Input: dimensioned drawing with shaded views. Units: mm. Origin: part minimum x, y, z. A direction names the side the tool comes from. Give positions to 0.01 mm unless a question says otherwise; leave off trailing zeros. Order: outer loops, then holes, each group sorted by start corner. A loop starts at its lowest first (then second) coordinate and runs counter-clockwise, first axis right, second up. Notation, with made-up numbers: (6, 71) - (55, 71) arc R14 ccw to (55, 85) - close; hole circle Ø1 at (9, 28.5). An arc over 180 degrees is marked (long way). Answer as CSV lines item,"result".
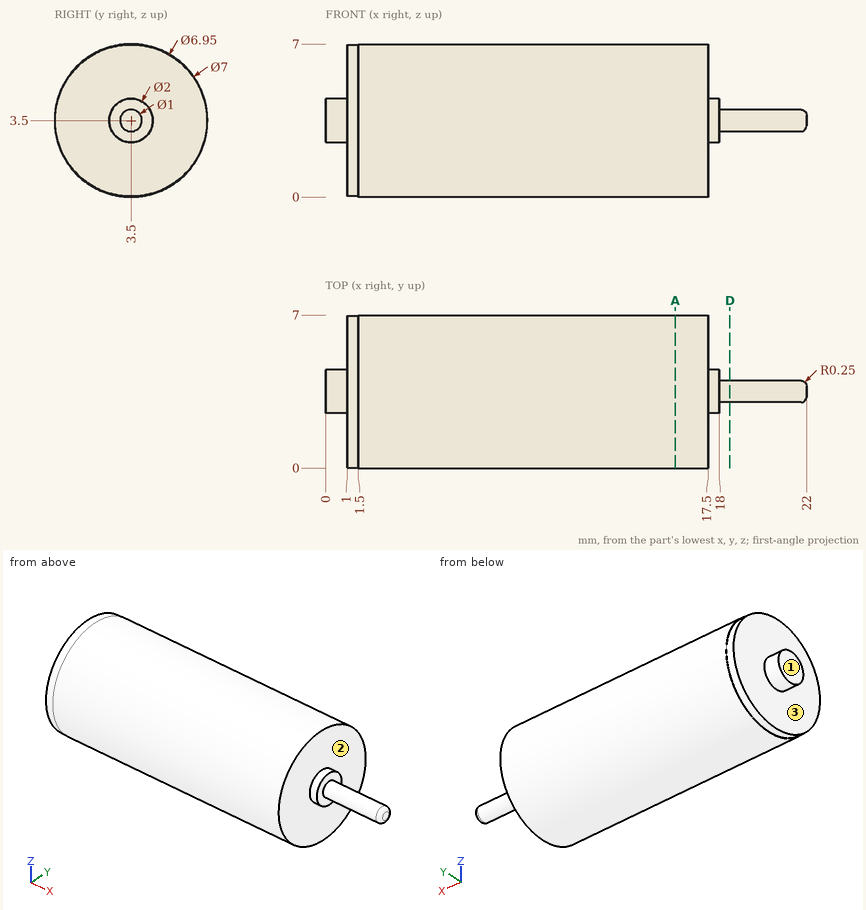
(1) Cut plane D-D (x = 18.5). Return loops of the section in (y, z).
Completed:
outline,"circle Ø1 at (3.5, 3.5)"
(2) Cut plane A-A (x = 16). Return loops of the section in (y, z), then the cut area to 3 significant figures.
Completed:
outline,"circle Ø7 at (3.5, 3.5)"
area,"38.5 mm²"
(3) Ray query, line 1 (X direction, y = 0.75, z = 2.5); line 2 (X direction, y = 4.25, z = 3); line 3 (Z direction, x = 9.25, y = 4.75). Return the intervals inside material, ascending. Write a range as from..to.
Completed:
line 1,"1..17.5"
line 2,"0..18"
line 3,"0.23..6.77"
(4) Contact query for flat-ended pins moving along their axis: pin 1 (4 mm diameter, centred on y = 4.5, z = 1, fed in from -X); pin 2 (1.5 mm diameter, centred on y = 6, z = 4.5, fed in from +X). Output: stop coordinate, or through.
Completed:
pin 1,"x = 0"
pin 2,"x = 17.5"
(5) Access query for the marked faces 1, 2 and 3. Directions: +Z, -Z, +X, -X, +Y, -Y. A direction counts if a zero-diameter tool reaches every point of the face in a straight line with its end or side. Return the directions, or none.
Completed:
face 1,"+Z, -Z, -X, +Y, -Y"
face 2,"+X"
face 3,"-X"
